Build history of the part. All positions in model axes, mm. Face numbers are marked on the shaded views. Give positions to 0.01 mm unless a question says otherwise; leave off trailing zeros. Loops run counter-clockwise (first coordinate to the right, second up) from the corner with the lowest first, then second, coordinate; pieces in that order, holes last. Notation, with made-up numbers: (75.25, 20) -> (120.25, 20) arc R23 ccw to (120.25, 56) -> close; hole circle Ø10 at (-32.5, -25.75). An arc over 180 degrees is marked (long way). Answer as a JSON object with one key per item and string values. Group by question number.
Q1. Band-saw the part on A-A, the plane y = -48.5. Write the cut outline in (x, z).
Q2. Wall check: probe 1 along Z at (x, y) = (29, -105); probe 2 along Z at (x, y) = (10, -107.5); probe 3 along X at (y, z) = (-80, 8). Give the ranges that are in metal, low to high. Write a range as from..to.
Q3. Drop flat-ended pins along their axis: pin 1 (9.5 mm diameter, centred on x = -30, y = -103, fed in from -Z); pin 2 (6 mm diameter, centred on x = -32, y = -82, fed in from +Z); pin 3 (1 mm diameter, centred on x = 14.5, y = -86.5, fed in from +Z). Give the stop position or say it passes through.
Q4. Two-plate mould, pull along X, no slides. Class the marked faces 1, 2 and 3: pulls with the +X half, pulls with the -X half, needs draft (parallel to the pull), parting line crosses it, or undercut.
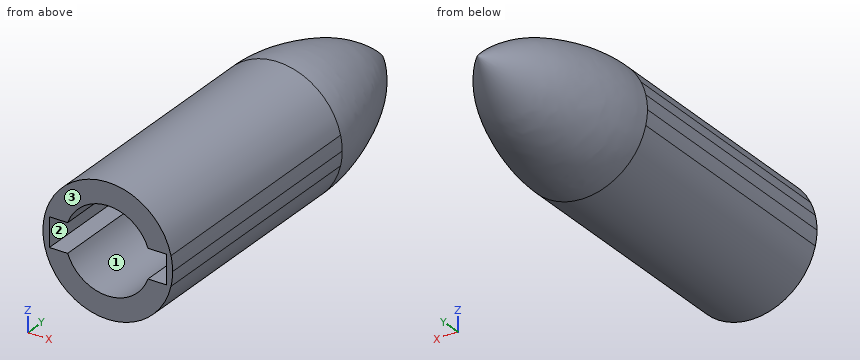
from build123d import *

# Parameters (mm, degrees)
BOSS_EXTRUDE1_DEPTH = 160


with BuildPart() as part:
    # Sketch1 → Boss-Extrude1 (new body)
    with BuildSketch(Plane(origin=(0, 0, 0), x_dir=(1, 0, 0), z_dir=(0, 1, 0))):
        with BuildLine():
            ThreePointArc((41, 0), (40.739454279, 4.61485266), (39.961128533, 9.171052632))
            Line((39.961128533, 9.171052632), (37.026014985, 9.171052632))
            Line((37.026014985, 9.171052632), (37.026014985, 0))
            Line((37.026014985, 0), (41, 0))
        make_face()
        with BuildLine():
            ThreePointArc((39.961128533, -9.171052632), (40.739454279, -4.61485266), (41, 0))
            Line((41, 0), (37.026014985, 0))
            Line((37.026014985, 0), (37.026014985, -9.171052632))
            Line((37.026014985, -9.171052632), (39.961128533, -9.171052632))
        make_face()
        with BuildLine():
            Line((-36.973985015, 0), (-41, 0))
            ThreePointArc((-41, 0), (-40.739454279, -4.61485266), (-39.961128533, -9.171052632))
            Line((-39.961128533, -9.171052632), (-36.973985015, -9.171052632))
            Line((-36.973985015, -9.171052632), (-36.973985015, 0))
        make_face()
        with BuildLine():
            Line((-25.394719798, -9.171052632), (-36.973985015, -9.171052632))
            Line((-36.973985015, -9.171052632), (-36.973985015, -17.717912748))
            ThreePointArc((-36.973985015, -17.717912748), (4.526915182, -40.74931949), (39.961128533, -9.171052632))
            Line((39.961128533, -9.171052632), (37.026014985, -9.171052632))
            Line((37.026014985, -9.171052632), (25.394719798, -9.171052632))
            ThreePointArc((25.394719798, -9.171052632), (0, -27), (-25.394719798, -9.171052632))
        make_face()
        with BuildLine():
            Line((-36.973985015, 9.171052632), (-39.961128533, 9.171052632))
            ThreePointArc((-39.961128533, 9.171052632), (-40.739454279, 4.61485266), (-41, 0))
            Line((-41, 0), (-36.973985015, 0))
            Line((-36.973985015, 0), (-36.973985015, 9.171052632))
        make_face()
        with BuildLine():
            ThreePointArc((39.961128533, 9.171052632), (0, 41), (-39.961128533, 9.171052632))
            Line((-39.961128533, 9.171052632), (-36.973985015, 9.171052632))
            Line((-36.973985015, 9.171052632), (-25.394719798, 9.171052632))
            ThreePointArc((-25.394719798, 9.171052632), (0, 27), (25.394719798, 9.171052632))
            Line((25.394719798, 9.171052632), (37.026014985, 9.171052632))
            Line((37.026014985, 9.171052632), (39.961128533, 9.171052632))
        make_face()
        with BuildLine():
            Line((-36.973985015, -9.171052632), (-39.961128533, -9.171052632))
            ThreePointArc((-39.961128533, -9.171052632), (-38.7042004, -13.527190078), (-36.973985015, -17.717912748))
            Line((-36.973985015, -17.717912748), (-36.973985015, -9.171052632))
        make_face()
    extrude(amount=-BOSS_EXTRUDE1_DEPTH)

    # Sketch2 → Revolve1 (revolve)
    with BuildSketch(Plane.XY):
        with BuildLine():
            Line((0, 0), (0, 99.064623465))
            add(Edge.make_bspline(
                [(0, 99.064623465), (11.435717322, 87.036046157), (23.647174069, 70.328206009), (36.388082529, 36.329625432), (40.969226805, 16.559428814), (41, 0)],
                knots=[0, 0, 0, 0, 0.458505426, 0.547537698, 1, 1, 1, 1], degree=3))
            Line((41, 0), (0, 0))
        make_face()
    revolve(axis=Axis((0, 0, 0), (0, 1, 0)))


solid = part.part
Worked answers:
{
 "1": {"outline": "circle Ø82 at (0, 0); hole (-36.97, -9.17) -> (-25.39, -9.17) arc R27 ccw to (25.39, -9.17) -> (37.03, -9.17) -> (37.03, 9.17) -> (25.39, 9.17) arc R27 ccw to (-25.39, 9.17) -> (-36.97, 9.17) -> close"},
 "2": {"probe 1": "-28.98..-9.17, 9.17..28.98", "probe 2": "-39.76..-25.08, 25.08..39.76", "probe 3": "-40.21..-36.97, 37.03..40.21"},
 "3": {"pin 1": "z = -32.3", "pin 2": "z = 28.98", "pin 3": "z = 38.54"},
 "4": {"face 1": "undercut", "face 2": "undercut", "face 3": "needs draft"}
}
